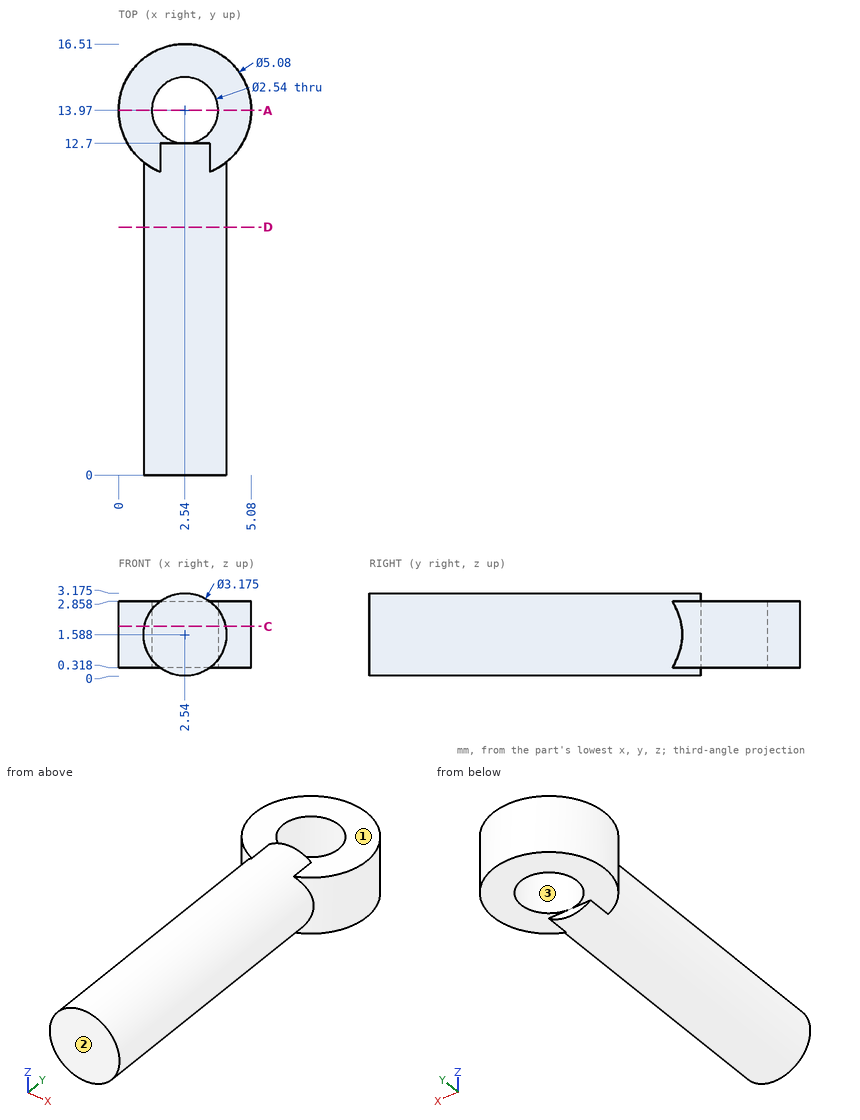
Part print with two shaded views. Sizes in mm from the minimum x, y, z corner. Round coordinates to 2 decimals unless told otherwise and drop trailing zeros. Order: outer loops, then holes, each group sorted by start corner. A loop starts at its lowest first (then second) coordinate and runs counter-clockwise, first axis right, second up. Notation, with made-up numbers: (76, 32.25) -> (118, 32.25) arc R14 cw to (118, 36.25) -> close; hole circle Ø4 at (63.25, -1). An arc over 180 degrees is marked (long way). Write each question's results on one line, items separated by ' | '.
1. Cut at A-A (y = 13.97). Give the cut face in (x, z).
Findings below:
outline: (0, 0.32) -> (1.27, 0.32) -> (1.27, 2.86) -> (0, 2.86) -> close; (3.81, 0.32) -> (5.08, 0.32) -> (5.08, 2.86) -> (3.81, 2.86) -> close
2. Cut at D-D (y = 9.5). Give the cut face in (x, z) (1 decimal).
Findings below:
outline: circle Ø3.2 at (2.5, 1.6)
3. Pull direction Y, two halves, no side cores. Call the marked faces 1, 2 and 3: pulls with the +Y half, pulls with the -Y half, needs draft (parallel to the pull), parting line crosses it, or undercut.
Findings below:
face 1: needs draft | face 2: pulls with the -Y half | face 3: undercut
4. Cut at C-C (z = 1.9). Give the cut face in (x, y).
Findings below:
outline: (0.98, 0) -> (4.1, 0) -> (4.1, 11.96) arc R2.54 ccw (long way) to (0.98, 11.96) -> close; hole circle Ø2.54 at (2.54, 13.97)
5. Flat gauge pins, fed straight in: P1, Ø2, axis at x = 3, y = 5, coming from the +Z side (1 decimal); P2, Ø2.5, axis at x = 1.5, y = 14, coming from the -Z side; P3, Ø1, axis at x = 1, z = 2.5, coming from the +Y side; P4, Ø3, axis at x = 4.5, y = 6.5, coming from the +Z side. Where does each tip first touch, or does it go through?
Findings below:
P1: stops at z = 3.2 | P2: stops at z = 0.32 | P3: stops at y = 16.29 | P4: stops at z = 3.11
6. Wall check: line 1 along X through (y, z) = (13.97, 1.15); line 2 along Z through (x, y) = (0.6, 13.25); line 3 along X through (y, z) = (1, 1.5) (1 decimal). Give the ranges that are in metal, low to high. Write a range as [from, to].
Findings below:
line 1: x = [0, 1.27], [3.81, 5.08] | line 2: z = [0.32, 2.86] | line 3: x = [1, 4.1]
